For this review, take the finished solid that the model builds, in its own axes (mm). Face numbers are marked on the shaded views. A direction names the side the tool comes from. Coordinates: 2 decimals unless noted, no trailing zeros. Loops run counter-clockwise (first coordinate to the right, second up) from the corner with the lowest first, then second, coordinate; pieces in that order, holes last. Notation, with made-up numbers: (-19.75, -1) - (21.25, -1) arc R27 cw to (21.25, 24) - close; hole circle Ø7 at (-31.5, 73.25). An arc over 180 degrees is marked (long way). Use one line per item in the form item = value. Start each with the question number.
1. Add section A-A on x = 42.3. Give the boundary of the cut face in (y, z) (3 decimals), and give its area (3 significant figures).
2. To check wall thickness, follow probe 1 along X at (y, z) = (10, 15.5); probe 2 along Z at (x, y) = (42, 6); probe 3 along X at (y, z) = (5, 16.5). State the ranges of each line that lie inside material, in increasing order.
3. Machinability: for the marked faces 1, 2, 3, 4 and 5, which of the approach directions +Z, -Z, +X, -X, +Y, -Y give a long, thin tool a straight path to every point of the face, cutting with its end or side? Answer none if there is none.
4. Add section B-B on y = 4. Give the boundary of the cut face in (x, z) (3 decimals), and give its area (3 significant figures).
5. Add section D-D on z = 0. Give the boundary of the cut face in (x, y), and give its area (3 significant figures).
6. Add section C-C on z = 15.8. Give the boundary of the cut face in (x, y) (3 decimals).
7. Draft analysis for pull direction X (two halves, no side actions). For the marked faces 6, 7 and 8, state which applies: +X half, -X half, draft (parallel to the pull), parting line (faces both ways), or undercut.
8. For pin 1 Ø10 at (x, z) = (-42.3, -15.8) entering from -Y; pin 2 Ø1.5 at (y, z) = (-13, -8.5) entering from +X; pin 3 Ø10 at (y, z) = (-13.5, 31.5) entering from -X, all flat-tipped, find the tip position at first contact; note any pin that passes through.
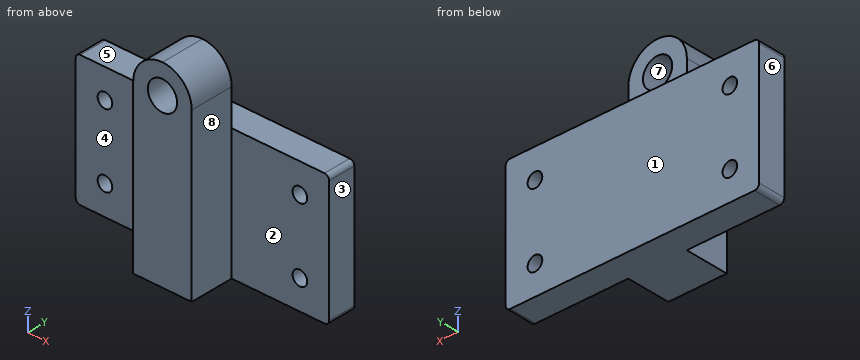
```python
from build123d import *

# Parameters (mm, degrees)
F0_W     = 25.4
F0_H     = 57
F0_R     = 3.175
F1_DEPTH = 12
F0_R_2   = 6.35
F2_DEPTH = 19.05


with BuildPart() as f1:
    # F0 (on Front) → F1 (new body)
    with BuildSketch(Plane.XZ):
        Rectangle(F0_W, F0_H)
        with BuildLine():
            Line((-12.7, 28.5), (-53, 28.5))
            ThreePointArc((-53, 28.5), (-54.4142135624, 27.9142135624), (-55, 26.5))
            Line((-55, 26.5), (-55, -26.5))
            ThreePointArc((-55, -26.5), (-54.4142135624, -27.9142135624), (-53, -28.5))
            Line((-53, -28.5), (-12.7, -28.5))
            Line((-12.7, -28.5), (-12.7, 28.5))
        make_face()
        with Locations((-42.3, -15.8)):
            Circle(F0_R, mode=Mode.SUBTRACT)
        with Locations((-42.3, 15.8)):
            Circle(F0_R, mode=Mode.SUBTRACT)
        with BuildLine():
            Line((53, 28.5), (12.7, 28.5))
            Line((12.7, 28.5), (12.7, -28.5))
            Line((12.7, -28.5), (53, -28.5))
            ThreePointArc((53, -28.5), (54.4142135624, -27.9142135624), (55, -26.5))
            Line((55, -26.5), (55, 26.5))
            ThreePointArc((55, 26.5), (54.4142135624, 27.9142135624), (53, 28.5))
        make_face()
        with Locations((42.3, -15.8)):
            Circle(F0_R, mode=Mode.SUBTRACT)
        with Locations((42.3, 15.8)):
            Circle(F0_R, mode=Mode.SUBTRACT)
    extrude(amount=-F1_DEPTH)

    # F0 (on Front) → F2 (join)
    with BuildSketch(Plane.XZ):
        Rectangle(F0_W, F0_H)
        with BuildLine():
            Line((-12.7, 44.3), (-12.7, 28.5))
            Line((-12.7, 28.5), (12.7, 28.5))
            Line((12.7, 28.5), (12.7, 44.3))
            ThreePointArc((12.7, 44.3), (0, 31.6), (-12.7, 44.3))
        make_face()
        with BuildLine():
            ThreePointArc((0, 57), (-8.9802561211, 53.2802561211), (-12.7, 44.3))
            ThreePointArc((-12.7, 44.3), (0, 31.6), (12.7, 44.3))
            ThreePointArc((12.7, 44.3), (8.9802561211, 53.2802561211), (0, 57))
        make_face()
        with Locations((0, 44.3)):
            Circle(F0_R_2, mode=Mode.SUBTRACT)
    extrude(amount=F2_DEPTH)


solid = f1.part
```
Conclusion:
q1.outline = (0, -28.5) - (12, -28.5) - (12, -18.975) - (0, -18.975) - close; (0, -12.625) - (12, -12.625) - (12, 12.625) - (0, 12.625) - close; (0, 18.975) - (12, 18.975) - (12, 28.5) - (0, 28.5) - close
q1.area = 532 mm^2
q2.probe_1 = -55 to -45.46, -39.14 to 39.14, 45.46 to 55
q2.probe_2 = -28.5 to -18.96, -12.64 to 12.64, 18.96 to 28.5
q2.probe_3 = -55 to -45.4, -39.2 to 39.2, 45.4 to 55
q3.face_1 = +Z, -Z, +X, -X, +Y
q3.face_2 = +Z, -Z, +X, -Y
q3.face_3 = +Z, -Z, +X, +Y, -Y
q3.face_4 = +Z, -Z, -X, -Y
q3.face_5 = +Z, +X, -X, +Y
q4.outline = (-55, -26.5) arc R2 ccw to (-53, -28.5) - (53, -28.5) arc R2 ccw to (55, -26.5) - (55, 26.5) arc R2 ccw to (53, 28.5) - (-53, 28.5) arc R2 ccw to (-55, 26.5) - close; hole circle Ø6.35 at (-42.3, -15.8); hole circle Ø6.35 at (-42.3, 15.8); hole circle Ø6.35 at (42.3, -15.8); hole circle Ø6.35 at (42.3, 15.8)
q4.area = 6,140 mm^2
q5.outline = (-55, 0) - (-12.7, 0) - (-12.7, -19.05) - (12.7, -19.05) - (12.7, 0) - (55, 0) - (55, 12) - (-55, 12) - close
q5.area = 1,800 mm^2
q6.outline = (-55, 0) - (-45.475, 0) - (-45.475, 12) - (-55, 12) - close; (-39.125, 0) - (-12.7, 0) - (-12.7, -19.05) - (12.7, -19.05) - (12.7, 0) - (39.125, 0) - (39.125, 12) - (-39.125, 12) - close; (45.475, 0) - (55, 0) - (55, 12) - (45.475, 12) - close
q7.face_6 = -X half
q7.face_7 = undercut
q7.face_8 = +X half
q8.pin_1 = 0
q8.pin_2 = 12.7
q8.pin_3 = -12.7
